from build123d import *

# Parameters (mm, degrees)
F1_DEPTH = 127
F2_DEPTH = 127
F4_DEPTH = 22.225
F5_DEPTH = 22.225


with BuildPart() as f1:
    # F0 (on Front) → F1 (new body)
    with BuildSketch(Plane.XZ):
        Polygon((-25.837215, 0.707869), (-44.887215, -31.042131), (-6.787215, -31.042131), (-6.787215, 32.457869), align=None)
    extrude(amount=F1_DEPTH)

    # F0 (on Front) → F2 (join)
    with BuildSketch(Plane.XZ):
        Polygon((-44.887215, 0), (-44.887215, -31.042131), (-25.837215, 0.707869), (-44.887215, 0.707869), align=None)
    extrude(amount=F2_DEPTH)

    # F3 (on face) → F4 (cut)
    with BuildSketch(Plane.XZ.offset(127)):
        Polygon((-44.887215, 0.707869), (-44.887215, -31.042131), (-25.837215, 0.707869), align=None)
    extrude(amount=-F4_DEPTH, mode=Mode.SUBTRACT)

    # F0 (on Front) → F5 (cut)
    with BuildSketch(Plane.XZ):
        Polygon((-44.887215, 0), (-44.887215, -31.042131), (-25.837215, 0.707869), (-44.887215, 0.707869), align=None)
    extrude(amount=F5_DEPTH, mode=Mode.SUBTRACT)


solid = f1.part
Geometry: final body of the model. Coordinates: model frame, mm. A direction names the side the tool comes from. Round coordinates to 2 decimals unless told otherwise and drop trailing zeros. Loops run counter-clockwise (first coordinate to the right, second up) from the corner with the lowest first, then second, coordinate; pieces in that order, holes last. Notation, with made-up numbers: M 58,-11.5 L 78,-11.5 A37 ccw 78,26.5 Z; hole C 18,51.5 d4. An arc over 180 degrees is marked long. Put each result on its own line as item: value. Start each with the question number.
(1) Section query B-B (x = -33.5). Return loops of the section in (y, z) (3 decimals).
(2) Section query C-C (y = -33). Return loops of the section in (x, z), then the cut area to 3 significant figures.
(3) Section query A-A (z = -13). Return loops of the section in (x, y) (3 decimals), then the cut area to 3 significant figures.
(4) Section query D-D (y = -19.5). Return loops of the section in (x, z), then the cut area to 3 significant figures.
(5) Contact query for flat-ended pins moving along their axis: pin 1 Ø8 at (x, y) = (-35.5, -41) entering from +Z; pin 2 Ø1.5 at (y, z) = (-16, 12.5) entering from -X. Output: stop coordinate, or through.
(6) Set-up query: faces 1 (the face through (-18, 0, -13)), 2 (the face through (-35, -63, 0.708)), 3 (the face through (-38, -22.225, -11)), 4 (the face through (-38, -104.775, -11)). Return all of +Z, -Z, +X, -X, +Y, -Y with unobstructed straight access to the full face (end or side cutting, diameter ignored); none if empty.
(7) Material intervals for line 1 along Z through (x, y) = (-26.5, -83); line 2 along X through (y, z) = (-92.5, 6.5); line 3 along X through (y, z) = (-12, 10), sorted ascending. Write a range as [from, to].
Findings below:
1. outline: M -127,-31.042 L 0,-31.042 L 0,-12.063 L -22.225,-12.063 L -22.225,0.708 L -104.775,0.708 L -104.775,-12.063 L -127,-12.063 Z
2. outline: M -44.89,-31.04 L -6.79,-31.04 L -6.79,32.46 L -25.84,0.71 L -44.89,0.71 Z
2. area: 1,510 mm2
3. outline: M -44.887,-104.775 L -34.062,-104.775 L -34.062,-127 L -6.787,-127 L -6.787,0 L -34.062,0 L -34.062,-22.225 L -44.887,-22.225 Z
3. area: 4,360 mm2
4. outline: M -44.89,-31.04 L -6.79,-31.04 L -6.79,32.46 Z
4. area: 1,210 mm2
5. pin 1: stops at z = 0.71
5. pin 2: stops at x = -19.21
6. face 1: +Z, -Z, +X, -X, +Y
6. face 2: +Z, -X, +Y, -Y
6. face 3: +Z, -X, +Y
6. face 4: +Z, -X, -Y
7. line 1: z = [-31.04, 0.71]
7. line 2: x = [-22.36, -6.79]
7. line 3: x = [-20.26, -6.79]
